Solid Edge part; units mm, degrees
sketch "Sketch1" plane through (0, 0, 0) normal (0, 0, -1) x (-1, 0, 0)
  line L0 (20.5, 70) -> (43.5, 70)
  line L1 (43.5, 70) -> (43.5, 82)
  line L2 (43.5, 82) -> (20.5, 82)
  line L3 (20.5, 82) -> (20.5, 70)
  line L4 (50.5, 70) -> (73.5, 70)
  line L5 (73.5, 70) -> (73.5, 82)
  line L6 (73.5, 82) -> (50.5, 82)
  line L7 (50.5, 82) -> (50.5, 70)
  circle A0 centre (2.5, 84.5) radius 1.75
  circle A1 centre (90.5, 84.5) radius 1.75
  circle A2 centre (2.5, 19.5) radius 1.75
  circle A3 centre (90.5, 19.5) radius 1.75
  line L8 (96, -0.5) -> (96, 87.5)
  arc A4 (96, 87.5) -> (93.5, 90) centre (93.5, 87.5) ccw
  line L9 (93.5, 90) -> (-0.5, 90)
  arc A5 (-0.5, 90) -> (-3, 87.5) centre (-0.5, 87.5) ccw
  line L10 (-3, 87.5) -> (-3, -0.5)
  arc A6 (-3, -0.5) -> (-0.5, -3) centre (-0.5, -0.5) ccw
  line L11 (-0.5, -3) -> (93.5, -3)
  arc A7 (96, -0.5) -> (93.5, -3) centre (93.5, -0.5) cw
extrude "Protrusion1" add sketch "Sketch1" along normal blind 10
sketch "Sketch2" plane through (-46.5, 43.5, 0) normal (0, 0, 1) x (1, 0, 0)
  line L0 (-49.5, -6.25) -> (-18.5, -6.25)
  line L1 (-18.5, -6.25) -> (-18.5, 23.75)
  line L2 (-18.5, 23.75) -> (-49.5, 23.75)
  line L3 (-49.5, 23.75) -> (-49.5, -6.25)
extrude "ExtrudedCutout_1" cut sketch "Sketch2" against normal blind 6
sketch "Sketch3" plane through (-46.5, 43.5, 0) normal (0, 0, 1) x (1, 0, 0)
  line L0 (-47.5, -44.5) -> (47.5, -44.5)
  line L1 (47.5, -44.5) -> (47.5, 44.5)
  line L2 (47.5, 44.5) -> (-47.5, 44.5)
  line L3 (-47.5, 44.5) -> (-47.5, -44.5)
extrude "ExtrudedCutout_3" cut sketch "Sketch3" against normal blind 8
sketch "Sketch4" plane through (-46.5, 43.5, -8) normal (0, 0, 1) x (1, 0, 0)
  line L0 (39.5, 44.5) -> (39.5, 40.5)
  arc A0 (39.5, 40.5) -> (43.5, 36.5) centre (43.5, 40.5) ccw
  line L1 (43.5, 36.5) -> (47.5, 36.5)
  line L2 (47.5, 36.5) -> (47.5, 44.5)
  line L3 (47.5, 44.5) -> (39.5, 44.5)
  line L4 (-47.5, -28) -> (-42.5, -28)
  arc A1 (-42.5, -28) -> (-40.5, -26) centre (-42.5, -26) ccw
  line L5 (-40.5, -26) -> (-40.5, -22.5)
  arc A2 (-40.5, -22.5) -> (-43, -20) centre (-43, -22.5) ccw
  line L6 (-43, -20) -> (-47.5, -20)
  line L7 (-47.5, -20) -> (-47.5, -28)
  line L8 (42.5, -27.5) -> (47.5, -27.5)
  line L9 (47.5, -27.5) -> (47.5, -20)
  line L10 (47.5, -20) -> (43, -20)
  arc A3 (43, -20) -> (40.5, -22.5) centre (43, -22.5) ccw
  line L11 (40.5, -22.5) -> (40.5, -25.5)
  arc A4 (42.5, -27.5) -> (40.5, -25.5) centre (42.5, -25.5) cw
  circle A5 centre (-44, 41) radius 1.75
  circle A6 centre (44, 41) radius 1.75
  circle A7 centre (44, -24) radius 1.75
  circle A8 centre (-44, -24) radius 1.75
  line L12 (-47.5, 36.5) -> (-43.5, 36.5)
  arc A9 (-43.5, 36.5) -> (-39.5, 40.5) centre (-43.5, 40.5) ccw
  line L13 (-39.5, 40.5) -> (-39.5, 44.5)
  line L14 (-39.5, 44.5) -> (-47.5, 44.5)
  line L15 (-47.5, 44.5) -> (-47.5, 36.5)
  dimension "D1" = 44
extrude "ExtrudedProtrusion_2" add sketch "Sketch4" along normal blind 5.8
sketch "Sketch5" plane through (-46.5, 43.5, -10) normal (0, 0, -1) x (-1, 0, 0)
  line L0 (-45.7321, 44) -> (-47.4641, 41)
  line L1 (-47.4641, 41) -> (-45.7321, 38)
  line L2 (-45.7321, 38) -> (-42.2679, 38)
  line L3 (-42.2679, 38) -> (-40.5359, 41)
  line L4 (-40.5359, 41) -> (-42.2679, 44)
  line L5 (-42.2679, 44) -> (-45.7321, 44)
  line L6 (42.2679, 44) -> (40.5359, 41)
  line L7 (40.5359, 41) -> (42.2679, 38)
  line L8 (42.2679, 38) -> (45.7321, 38)
  line L9 (45.7321, 38) -> (47.4641, 41)
  line L10 (47.4641, 41) -> (45.7321, 44)
  line L11 (45.7321, 44) -> (42.2679, 44)
  line L12 (-45.7321, -21) -> (-47.4641, -24)
  line L13 (-47.4641, -24) -> (-45.7321, -27)
  line L14 (-45.7321, -27) -> (-42.2679, -27)
  line L15 (-42.2679, -27) -> (-40.5359, -24)
  line L16 (-40.5359, -24) -> (-42.2679, -21)
  line L17 (-42.2679, -21) -> (-45.7321, -21)
  line L18 (42.2679, -21) -> (40.5359, -24)
  line L19 (40.5359, -24) -> (42.2679, -27)
  line L20 (42.2679, -27) -> (45.7321, -27)
  line L21 (45.7321, -27) -> (47.4641, -24)
  line L22 (47.4641, -24) -> (45.7321, -21)
  line L23 (45.7321, -21) -> (42.2679, -21)
extrude "ExtrudedCutout_4" cut sketch "Sketch5" against normal blind 3.5
sketch "Sketch6" plane through (-46.5, 43.5, -10) normal (0, 0, -1) x (-1, 0, 0)
  circle A0 centre (17.5, 17.5) radius 1.6
  circle A1 centre (-17.5, -17.5) radius 1.6
  circle A2 centre (17.5, -17.5) radius 1.6
  circle A3 centre (-17.5, 17.5) radius 1.6
extrude "ExtrudedCutout_5" cut sketch "Sketch6" against normal blind 2
sketch "Sketch7" plane through (-46.5, 43.5, -8) normal (0, 0, 1) x (0, -1, 0)
  circle A0 centre (-17.5, -17.5) radius 3
  circle A1 centre (-17.5, 17.5) radius 3
  circle A2 centre (17.5, 17.5) radius 3
  circle A3 centre (17.5, -17.5) radius 3
extrude "ExtrudedCutout_6" cut sketch "Sketch7" against normal blind 0.5
fillet "Round_1" radius 1 8 edges at (-46.5, 90, -10) (2.2678, 89.2678, -10) (3, 43.5, -10) (2.2678, -2.2678, -10) (-46.5, -3, -10) (-95.2678, -2.2678, -10) (-96, 43.5, -10) (-95.2678, 89.2678, -10)
The listing builds one solid part. Answer for the finished solid, in the listing's coordinates (mm). A direction names the side the tool comes from. Coordinates: 2 decimals unless noted, no trailing zeros. Write each loop counter-clockwise with the first axis right and the second up, starting at its lowest first coordinate (ties: lowest second). Pieces come first, ordered by that corner, then holes. Notation, with made-up numbers: (41.5, 64) - (97.5, 64) arc R22 ccw to (97.5, 85) - close; hole circle Ø8 at (-13, -19.75). An arc over 180 degrees is marked (long way). Answer as CSV lines item,"result".
1. A tool of negligible diameter and unlimited length cuts with its end or side. For faces 1 (the flat face through (-87.9, 86, -8.3)), 2 (the cylindrical face through (-2.728, 17.765, -4.38)), 3 (the flat face through (-62.7, 24.7, -8.5)), from which of +Z, -Z, +X, -X, +Y, -Y can it reach the whole face along a straight path? Write none if from no direction.
Computed values:
face 1,"-Z"
face 2,"+Z, -Z"
face 3,"+Z"
2. Given P1, Ø6.5, axis at x = -63.5, y = 26.5, coming from the +Z side; P2, Ø0.6, axis at x = -95.5, z = -4, coming from the -Y side; P3, Ø1.8, axis at x = -30, y = 62.5, coming from the +Z side, each flat-ended and moving along its own axis, determine where each tip first touches the part or whether it passes through.
Computed values:
P1,"stops at z = -8"
P2,"stops at y = -2.33"
P3,"stops at z = -8.5"
3. Find section D-D (y = 61). Give the vertices of the cut face in (x, z), plus the area to 3 significant figures.
Computed values:
outline,"(-96, -9) arc R1 ccw to (-95, -10) - (-65.6, -10) - (-65.6, -8.5) - (-67, -8.5) - (-67, -8) - (-94, -8) - (-94, -6) - (-96, -6) - close; (-62.4, -10) - (-30.6, -10) - (-30.6, -8.5) - (-32, -8.5) - (-32, -8) - (-61, -8) - (-61, -8.5) - (-62.4, -8.5) - close; (-27.4, -10) - (2, -10) arc R1 ccw to (3, -9) - (3, 0) - (1, 0) - (1, -8) - (-26, -8) - (-26, -8.5) - (-27.4, -8.5) - close"
area,"202 mm²"
4. Find section A-A (y = 26). Give the vertices of the cut face in (x, z), plus the area to 3 significant figures.
Computed values:
outline,"(-96, -9) arc R1 ccw to (-95, -10) - (-65.6, -10) - (-65.6, -8.5) - (-67, -8.5) - (-67, -8) - (-94, -8) - (-94, 0) - (-96, 0) - close; (-62.4, -10) - (-30.6, -10) - (-30.6, -8.5) - (-32, -8.5) - (-32, -8) - (-61, -8) - (-61, -8.5) - (-62.4, -8.5) - close; (-27.4, -10) - (2, -10) arc R1 ccw to (3, -9) - (3, 0) - (1, 0) - (1, -8) - (-26, -8) - (-26, -8.5) - (-27.4, -8.5) - close"
area,"214 mm²"
5. Find section B-B (x = -40). Give the vertices of the cut face in (y, z).
Computed values:
outline,"(-3, -9) arc R1 ccw to (-2, -10) - (70, -10) - (70, -8) - (-1, -8) - (-1, 0) - (-3, 0) - close; (82, -10) - (89, -10) arc R1 ccw to (90, -9) - (90, 0) - (88, 0) - (88, -8) - (82, -8) - close"
6. Find section C-C (x = -29). Give the number of separate pieces and of enclosed holes in the cut face, plus the area to 3 significant figures.
Computed values:
separate pieces,"4"
enclosed holes,"0"
area,"178 mm²"
7. Straight lines are drawn through the part: line 1 (Y direction, x = -29, z = -9.2); line 2 (Y direction, x = -1.5, z = -8.75); line 3 (X direction, y = 67, z = -7.75). For each, find the intervals that lie inside material, in ascending order. Write a range as [from, to].
Computed values:
line 1,"y = [-2.98, 24.4], [27.6, 59.4], [62.6, 70], [82, 89.98]"
line 2,"y = [-3, 16.5], [22.5, 81.5], [87.5, 90]"
line 3,"x = [-96, -94], [1, 3]"
8. Determine the mould class of faces 4 (the flat face through (-47, 90, -4)), 5 (the flat face through (-46, 44, -10)), 6 (the cylindrical face through (-63.9, 64, -8.2)) for opening direction Y: +Y half, -Y half, draft (parallel to the pull), parting line (faces both ways), or undercut.
Computed values:
face 4,"+Y half"
face 5,"draft"
face 6,"undercut"
